Build history of the part. All positions in model axes, mm. A direction names the side the tool comes from. Give positions to 0.01 mm unless a question says otherwise; leave off trailing zeros. Write each loop counter-clockwise with the first axis right and the second up, starting at its lowest first coordinate (ties: lowest second). Pieces come first, ordered by that corner, then holes. Notation, with made-up numbers: M 38,0 L 87,0 A15 ccw 87,17 Z; hole C -14.5,69.5 d4. An arc over 180 degrees is marked long. One line per item, written item: value. Start each with the question number.
Autodesk Inventor part; units mm, degrees
ref_plane "РабПлоскость2" through (1941.2464, 6.5, -14) normal (0, 0, 1) x (1, 0, 0)
ref_plane "YZ Plane" through (0, 0, 0) normal (1, 0, 0) x (0, 1, 0)
ref_plane "XZ Plane" through (0, 0, 0) normal (0, 1, 0) x (-1, 0, 0)
ref_plane "РабПлоскость1" through (1955.2464, 20.5, -10) normal (0, 0, 1) x (1, 0, 0)
sketch "Эскиз1" plane through (1955.2464, 20.5, -10) normal (0, 0, 1) x (1, 0, 0)
  circle A0 centre (0, 0) radius 14
  circle A1 centre (0, 0) radius 12.25
  point P0 (-1955.2464, -20.5)
  dimension "d0" = 28
  dimension "d1" = 24.5
ref_plane "РабПлоскость2" through (1941.2464, 6.5, -14) normal (0, 0, 1) x (1, 0, 0)
extrude "Выдавливание1" add sketch "Эскиз1" against normal up to surface (4 mm away)
sketch "Эскиз2" plane through (1955.2464, 20.5, -10) normal (0, 0, 1) x (1, 0, 0)
  circle A0 centre (0, 0) radius 14
  point P0 (-1955.2464, -20.5)
extrude "Выдавливание2" add sketch "Эскиз2" against normal blind 2.5
sketch "Эскиз3" plane through (1955.2464, 20.5, -12.5) normal (0, 0, -1) x (-1, 0, 0)
  circle A0 centre (0, 0) radius 2
  point P0 (1955.2464, -20.5)
  dimension "d6" = 4
sketch "Эскиз4" plane through (1955.2464, 20.5, -10) normal (0, 0, 1) x (1, 0, 0)
  circle A0 centre (0, 0) radius 2
  point P0 (-1955.2464, -20.5)
  dimension "d9" = 4
extrude "Выдавливание4" cut sketch "Эскиз4" against normal blind 2
properties part number "крышка"
1) Drop flat-ended pins along their axis: P1, Ø2.5, axis at x = 1955.25, y = 20.5, coming from the +Z side; P2, Ø1, axis at x = 1951.5, z = -13.5, coming from the +Y side; P3, Ø1.5, axis at x = 1962, y = 20, coming from the -Z side. Give the stop position or say it passes through.
2) Mould opens along X. For faces 4 (the face through (1955, 21, -12)), 5 (the face through (1941.26, 21.12, -11.97)), 6 (the face through (1955, 8, -14)) say: released by +X, released by -X, zero draft, split by the parting line, or undercut.
3) Band-saw the part on B-B (z = -13.3). List the corners of the cut face in (x, y).
4) Band-saw the part on D-D (y = 23.75). List the corners of the cut face in (x, z).
5) Probe line 1 along Z through (x, y) = (1948, 25.5); line 2 along X through (y, z) = (25, -12.9); line 3 along Y through (x, z) = (1946.75, -13). List the from-to ranges inside material, lowest first. Write a range as from..to.
6) Band-saw the part on A-A (y = 20.5). List the corners of the cut face in (x, z), then the cut area to 4 significant figures.
7) Band-saw the part on C-C (x = 1965.75). List the corners of the cut face in (y, z).
8) Tool access for faces 1 (the face through (1943.01, 21.04, -13.24)), 2 (the face through (1957.154, 21.101, -10.986)), 3 (the face through (1958, 21, -10)): list every direction of +Z, -Z, +X, -X, +Y, -Y with a clear straight run to the whole face (end or side of a thin tool).
Model answer:
1. P1: stops at z = -12
1. P2: stops at y = 34.12
1. P3: stops at z = -12.5
2. face 4: undercut
2. face 5: split by the parting line
2. face 6: zero draft
3. outline: C 1955.25,20.5 d28; hole C 1955.25,20.5 d24.5
4. outline: M 1941.63,-14 L 1943.44,-14 L 1943.44,-12.5 L 1967.06,-12.5 L 1967.06,-14 L 1968.86,-14 L 1968.86,-10 L 1941.63,-10 Z
5. line 1: z = -12.5..-10
5. line 2: x = 1941.99..1943.85, 1966.64..1968.5
5. line 3: y = 9.37..11.68, 29.32..31.63
6. outline: M 1941.25,-14 L 1943,-14 L 1943,-12.5 L 1967.5,-12.5 L 1967.5,-14 L 1969.25,-14 L 1969.25,-10 L 1957.25,-10 L 1957.25,-12 L 1953.25,-12 L 1953.25,-10 L 1941.25,-10 Z
6. area: 67.25 mm²
7. outline: M 11.24,-14 L 14.2,-14 L 14.2,-12.5 L 26.8,-12.5 L 26.8,-14 L 29.76,-14 L 29.76,-10 L 11.24,-10 Z
8. face 1: -Z
8. face 2: +Z
8. face 3: +Z, +X, -X, +Y, -Y
